from build123d import *

# Parameters (mm, degrees)
SKETCH_1_R          = 2.95
EXTRUDE_1_DEPTH     = 2.7
SKETCH_2_R          = 1.25
EXTRUDE_2_DEPTH     = 20
SKETCH_3_R          = 1
EXTRUDE_3_DEPTH     = 4
CUT_EXTRUDE_1_DEPTH = 2
FILLET_1_R          = 0.2


with BuildPart() as part:
    # 草图1 → 凸台-拉伸1 (new body)
    with BuildSketch(Plane(origin=(0, 0, 0), x_dir=(1, 0, 0), z_dir=(0, 1, 0))):
        Circle(SKETCH_1_R)
    extrude(amount=EXTRUDE_1_DEPTH)

    # 草图2 → 凸台-拉伸2 (add)
    with BuildSketch(Plane(origin=(0, 2.7, 0), x_dir=(1, 0, 0), z_dir=(0, 1, 0))):
        Circle(SKETCH_2_R)
    extrude(amount=EXTRUDE_2_DEPTH)

    # 草图3 → 凸台-拉伸3 (add)
    with BuildSketch(Plane(origin=(0, 22.7, 0), x_dir=(1, 0, 0), z_dir=(0, 1, 0))):
        Circle(SKETCH_3_R)
    extrude(amount=EXTRUDE_3_DEPTH)

    # 草图4 → 切除-拉伸1 (cut)
    with BuildSketch(Plane.XZ):
        Polygon((2.247285488, -0.53201623), (1.584382314, 1.680198207), (-0.662903174, 2.212214437), (-2.247285488, 0.53201623), (-1.584382314, -1.680198207), (0.662903174, -2.212214437), align=None)
    extrude(amount=-CUT_EXTRUDE_1_DEPTH, mode=Mode.SUBTRACT)

    # 圆角1
    fillet_1_edges = [part.edges().sort_by_distance(p)[0] for p in [
        (-1, 26.7, 0),
        (-2.95, 0, 0),
        (-2.95, 2.7, 0),
    ]]
    fillet(fillet_1_edges, radius=FILLET_1_R)


solid = part.part
CAD build for the part. Positions are in the model's coordinates, mm. A direction names the side the tool comes from. Round coordinates to 2 decimals unless told otherwise and drop trailing zeros. Loops run counter-clockwise (first coordinate to the right, second up) from the corner with the lowest first, then second, coordinate; pieces in that order, holes last. Notation, with made-up numbers: M -22,36.25 L -13,36.25 A30 ccw -13,73.25 Z; hole C -10,0.25 d8. An arc over 180 degrees is marked long. One line per question, with ' | ' between items. Start each with the question number.
Item 1: Pin check, flat tips, straight feed: pin 1 Ø1.3 at (x, z) = (0.5, 0) entering from -Y; pin 2 Ø1.5 at (y, z) = (3, 2.5) entering from +X. Stop position of each tip, or through.
Item 2: Cut at A-A, the plane y = 10. Write the cut outline in (x, z).
Item 3: Cut at C-C, the plane y = 23. Write the cut outline in (x, z).
Item 4: Cut at B-B, the plane x = 0. Write the cut outline in (y, z), plus the area to 3 significant figures.
Item 5: Two-plate mould, pull along Z, no slides. Class faces 4 (the flat face through (0, 26.7, 0)), 5 (the flat face through (1.444, 0.986, -1.384)), 6 (the flat face through (1.92, 0.99, 0.56)), 7 (the cylindrical face through (-0.27, 12.56, 1.22)): pulls with the +Z half, pulls with the -Z half, needs draft (parallel to the pull), parting line crosses it, or undercut.
Item 6: Wall check: line 1 (Z direction, x = -0.1, y = 23.75); line 2 (Y direction, x = -2.45, z = -0.2); line 3 (Z direction, x = 0.05, y = 18.25). Give the ranges that are in metal, low to high.
Item 7: Which spindle directions (+Z, -Z, +X, -X, +Y, -Y) get a long thin tool onto all of the face, cutting with end or side? Do faces 1 (the flat face through (-1.444, 0.986, 1.384)), 2 (the cylindrical face through (0, 25, 1)), 3 (the cylindrical face through (-2.947, 1.334, -0.13)). Say none if no direction does.
Responses:
1) pin 1: stops at y = 2 | pin 2: stops at x = 2.25
2) outline: C 0,0 d2.5
3) outline: C 0,0 d2
4) outline: M 0,-2.75 A0.2 ccw 0.2,-2.95 L 2.5,-2.95 A0.2 ccw 2.7,-2.75 L 2.7,-1.25 L 22.7,-1.25 L 22.7,-1 L 26.5,-1 A0.2 ccw 26.7,-0.8 L 26.7,0.8 A0.2 ccw 26.5,1 L 22.7,1 L 22.7,1.25 L 2.7,1.25 L 2.7,2.75 A0.2 ccw 2.5,2.95 L 0.2,2.95 A0.2 ccw 0,2.75 L 0,2.06 L 2,2.06 L 2,-2.06 L 0,-2.06 Z | area: 65.7 mm²
5) face 4: needs draft | face 5: undercut | face 6: undercut | face 7: parting line crosses it
6) line 1: z = -0.99 to 0.99 | line 2: y = 0 to 2.7 | line 3: z = -1.25 to 1.25
7) face 1: -Y | face 2: +Y | face 3: +Y, -Y
